Autodesk Inventor part; units mm, degrees
ref_plane "YZ Plane" through (0, 0, 0) normal (1, 0, 0) x (0, 1, 0)
ref_plane "XZ Plane" through (0, 0, 0) normal (0, 1, 0) x (-1, 0, 0)
ref_plane "XY Plane" through (0, 0, 0) normal (0, 0, 1) x (1, 0, 0)
sketch "Sketch1" plane through (0, 0, 0) normal (0, 0, 1) x (1, 0, 0)
  circle A0 centre (0, 0) radius 114.3
  line L0 (7.6256, 0) -> (3.8128, -6.604)
  line L1 (3.8128, -6.604) -> (-3.8128, -6.604)
  line L2 (-3.8128, -6.604) -> (-7.6256, 0)
  line L3 (-7.6256, 0) -> (-3.8128, 6.604)
  line L4 (-3.8128, 6.604) -> (3.8128, 6.604)
  line L5 (3.8128, 6.604) -> (7.6256, 0)
  circle A1 centre (0, 101.6) radius 5.2705
  dimension "d0" = 228.6
  dimension "d1" = 13.208
  dimension "d2" = 10.541
  dimension "d5" = 101.6
extrude "Extrusion1" add sketch "Sketch1" along normal mid plane 12.7
sketch "Sketch4" plane through (0, 0, 6.35) normal (0, 0, 1) x (1, 0, 0)
  circle A0 centre (0, 0) radius 114.3
  line L0 (-38.1, 107.7631) -> (-38.1, -107.7631)
  line L1 (38.1, 107.7631) -> (38.1, -107.7631)
  arc A1 (-38.1, 107.7631) -> (-38.1, -107.7631) centre (0, 0) ccw
  arc A2 (38.1, -107.7631) -> (38.1, 107.7631) centre (0, 0) ccw
  dimension "d18" = 38.1
  dimension "d19" = 38.1
extrude "Extrusion4" cut sketch "Sketch4" against normal through all contours A0 L1 | L0 A0
sketch "Sketch2" plane through (0, 0, 6.35) normal (0, 0, 1) x (1, 0, 0)
  circle A0 centre (-63.5, 0) radius 25.4
  circle A1 centre (-31.75, -54.9926) radius 25.4
  circle A2 centre (31.75, -54.9926) radius 25.4
  circle A3 centre (63.5, 0) radius 25.4
  circle A4 centre (31.75, 54.9926) radius 25.4
  circle A5 centre (-31.75, 54.9926) radius 25.4
  point P0 (0, 0)
  dimension "d6" = 50.8
  dimension "d7" = 63.5
  dimension "d10" = 360
properties part number "driveForPiston-8-inV03" material "PET Plastic"
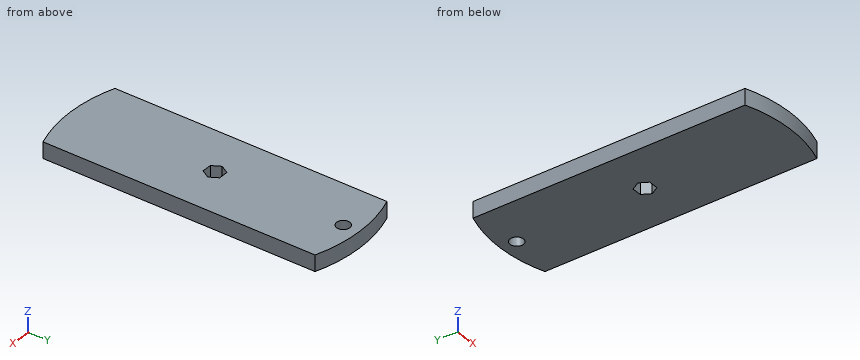
The listing builds one solid part. Answer for the finished solid, in the listing's coordinates (mm). Round coordinates to 2 decimals unless told otherwise and drop trailing zeros. Write each loop counter-clockwise with the first axis right and the second up, starting at its lowest first coordinate (ties: lowest second). Pieces come first, ordered by that corner, then holes. Notation, with made-up numbers: (29.5, 46) -> (63.5, 46) arc R10 ccw to (63.5, 55) -> close; hole circle Ø11 at (73.25, 11). An arc over 180 degrees is marked (long way). Answer as a JSON object with one key per item and string values. Group by question number.
Q1. Section A-A (y = 101.6) is taken. Write down the section's boundary in (x, z).
Q2. Section D-D (y = 4.5) is taken. Write down the section's boundary in (x, z), plus the area to 3 significant figures.
Q3. Each of these flat-tipped pins is pushed along its axis until it touches: pin 1 Ø4 at (x, z) = (-9.5, 3) entering from +Y; pin 2 Ø4 at (x, z) = (-6.5, 5) entering from +Y; pin 3 Ø6 at (x, z) = (-25.5, 2) entering from +Y; pin 4 Ø9.5 at (x, y) = (0, 101.6) entering from +Z. Where does it stop, or does it pass through?
Q4. Straight lines are drawn through the part: line 1 along Y through (x, z) = (0, 0); line 2 along Y through (x, z) = (1, -2.5); line 3 along X through (y, z) = (98, 4). For each, find the intervals that lie inside material, in ascending order.
Q5. Section C-C (z = -0.5) is taken. Write down the section's boundary in (x, y).
Q6. Section B-B (x = 0) is taken. Write down the section's boundary in (y, z).
Check values:
{
 "1": {"outline": "(-38.1, -6.35) -> (-5.27, -6.35) -> (-5.27, 6.35) -> (-38.1, 6.35) -> close; (5.27, -6.35) -> (38.1, -6.35) -> (38.1, 6.35) -> (5.27, 6.35) -> close"},
 "2": {"outline": "(-38.1, -6.35) -> (-5.03, -6.35) -> (-5.03, 6.35) -> (-38.1, 6.35) -> close; (5.03, -6.35) -> (38.1, -6.35) -> (38.1, 6.35) -> (5.03, 6.35) -> close", "area": "840 mm^2"},
 "3": {"pin 1": "y = 114.05", "pin 2": "y = 114.21", "pin 3": "y = 112.06", "pin 4": "through"},
 "4": {"line 1": "-114.3 to -6.6, 6.6 to 96.33, 106.87 to 114.3", "line 2": "-114.3 to -6.6, 6.6 to 96.43, 106.77 to 114.3", "line 3": "-38.1 to -3.85, 3.85 to 38.1"},
 "5": {"outline": "(-38.1, -107.76) arc R114.3 ccw to (38.1, -107.76) -> (38.1, 107.76) arc R114.3 ccw to (-38.1, 107.76) -> close; hole (-7.63, 0) -> (-3.81, -6.6) -> (3.81, -6.6) -> (7.63, 0) -> (3.81, 6.6) -> (-3.81, 6.6) -> close; hole circle Ø10.54 at (0, 101.6)"},
 "6": {"outline": "(-114.3, -6.35) -> (-6.6, -6.35) -> (-6.6, 6.35) -> (-114.3, 6.35) -> close; (6.6, -6.35) -> (96.33, -6.35) -> (96.33, 6.35) -> (6.6, 6.35) -> close; (106.87, -6.35) -> (114.3, -6.35) -> (114.3, 6.35) -> (106.87, 6.35) -> close"}
}
